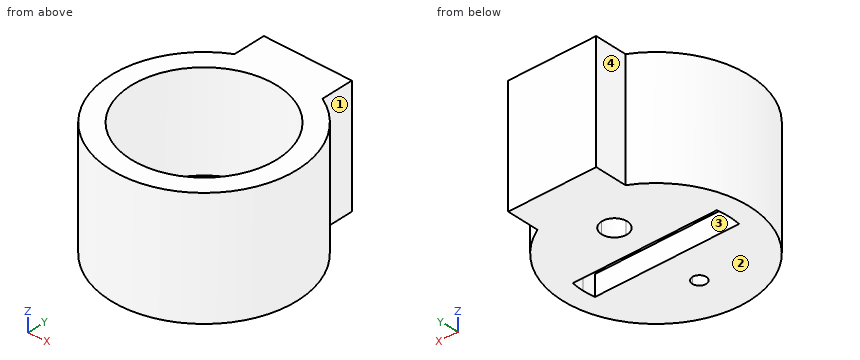
from build123d import *

# Parameters (mm, degrees)
F0_W     = 330
F0_H     = 300
F1_DEPTH = 110
F2_R     = 68.5
F3_DEPTH = 90.8
F5_DEPTH = 19.201
F2_W     = 330
F2_H     = 300
F2_R_2   = 87.5
F6_DEPTH = 110.001
F8_DEPTH = 110


with BuildPart() as f1:
    # F0 (on Top) → F1 (new body)
    with BuildSketch(Plane.XY):
        Rectangle(F0_W, F0_H)
    extrude(amount=-F1_DEPTH)

    # F2 (on Top) → F3 (cut)
    with BuildSketch(Plane.XY):
        Circle(F2_R)
    extrude(amount=-F3_DEPTH, mode=Mode.SUBTRACT)

    # F4 (on face) → F5 (cut, through all)
    with BuildSketch(Plane.XY.offset(-90.8)):
        with BuildLine():
            Line((0, -11.5), (0, 0))
            Line((0, 0), (0, 11.5))
            Line((0, 11.5), (-67.5277720645, 11.5))
            ThreePointArc((-67.5277720645, 11.5), (-68.5, 0), (-67.5277720645, -11.5))
            Line((-67.5277720645, -11.5), (0, -11.5))
        make_face()
        with BuildLine():
            Line((0, 11.5), (0, 0))
            Line((0, 0), (0, -11.5))
            Line((0, -11.5), (67.5277720645, -11.5))
            ThreePointArc((67.5277720645, -11.5), (68.2565102625, -5.7705118308), (68.5, 0))
            ThreePointArc((68.5, 0), (68.2565102625, 5.7705118308), (67.5277720645, 11.5))
            Line((67.5277720645, 11.5), (0, 11.5))
        make_face()
        with BuildLine():
            ThreePointArc((12, 43), (-8.4852813742, 51.4852813742), (0, 31))
            ThreePointArc((0, 31), (8.4852813742, 34.5147186258), (12, 43))
        make_face()
        with BuildLine():
            ThreePointArc((6.5, -45), (4.5961940777, -40.4038059223), (0, -38.5))
            ThreePointArc((0, -38.5), (-4.5961940777, -49.5961940777), (6.5, -45))
        make_face()
    extrude(amount=-F5_DEPTH, mode=Mode.SUBTRACT)

    # F2 (on Top) → F6 (cut, through all)
    with BuildSketch(Plane.XY):
        Rectangle(F2_W, F2_H)
        Circle(F2_R_2, mode=Mode.SUBTRACT)
    extrude(amount=-F6_DEPTH, mode=Mode.SUBTRACT)

    # F7 (on face) → F8 (join)
    with BuildSketch(Plane(origin=(0, 0, -110), x_dir=(1, 0, 0), z_dir=(0, 0, -1))):
        with BuildLine():
            ThreePointArc((41.25, -77.1666216703), (0, -87.5), (-41.25, -77.1666216703))
            Line((-41.25, -77.1666216703), (-41.25, -107.5))
            Line((-41.25, -107.5), (41.25, -107.5))
            Line((41.25, -107.5), (41.25, -77.1666216703))
        make_face()
    extrude(amount=-F8_DEPTH)


solid = f1.part
Design review of the part built by this model. Coordinates are the model's own, in mm. Face numbers are marked on the shaded views. Round coordinates to 2 decimals unless told otherwise and drop trailing zeros. Write each loop counter-clockwise with the first axis right and the second up, starting at its lowest first coordinate (ties: lowest second). Pieces come first, ordered by that corner, then holes. Notation, with made-up numbers: (9.25, -29) - (20.25, -29) arc R20 ccw to (20.25, -5) - close; hole circle Ø2 at (1.5, 57.25). An arc over 180 degrees is marked (long way). Use a Markdown table: item, result. Add a question column.
1. We need section C-C (z = -7.5). State the section outline as (x, y) points.
2. We need section D-D (y = -56). State the section outline as (x, z) points.
3. We need section B-B (y = -7). State the section outline as (x, z) points.
4. Wall thickness on probe 1 along Y at (x, z) = (0, -105.5); probe 2 along Y at (x, z) = (0, -36); probe 3 along Z at (x, y) = (37.5, -28.5): over which ranges is each line inside the solid? List them lowest first.
5. Clearance check with flat-ended pins moving along their axes: pin 1 (21 mm diameter, centred on x = 31, z = -101.5, fed in from -Y); pin 2 (5 mm diameter, centred on x = -31.5, z = -33, fed in from -Y); pin 3 (10 mm diameter, centred on x = 58, z = -33, fed in from +Y); pin 4 (10.5 mm diameter, centred on x = 0, y = -45, fed in from -Z). State where each tip first meets the part, or that it passes through.
6. Mouldability with a two-part tool opening along X and no side actions: class the marked faces 1, 2, 3 and 4 as +X half, -X half, draft (parallel to the pull), parting line (faces both ways), or undercut.
7. We need section A-A (z = -98). State the section outline as (x, y) points.
Output:
| question | item | result |
|---|---|---|
| 1 | outline | (-41.25, 77.17) arc R87.5 ccw (long way) to (41.25, 77.17) - (41.25, 107.5) - (-41.25, 107.5) - close; hole circle Ø137 at (0, 0) |
| 2 | outline | (-67.23, -110) - (67.23, -110) - (67.23, 0) - (39.45, 0) - (39.45, -90.8) - (-39.45, -90.8) - (-39.45, 0) - (-67.23, 0) - close |
| 3 | outline | (-87.22, -110) - (-68.14, -110) - (-68.14, 0) - (-87.22, 0) - close; (68.14, -110) - (87.22, -110) - (87.22, 0) - (68.14, 0) - close |
| 4 | probe 1 | y = -87.5 to -51.5, -38.5 to -11.5, 11.5 to 31, 55 to 107.5 |
| 4 | probe 2 | y = -87.5 to -68.5, 68.5 to 107.5 |
| 4 | probe 3 | z = -110 to -90.8 |
| 5 | pin 1 | stops at y = -85.06 |
| 5 | pin 2 | stops at y = -82.55 |
| 5 | pin 3 | stops at y = 69.62 |
| 5 | pin 4 | passes through |
| 6 | face 1 | +X half |
| 6 | face 2 | draft |
| 6 | face 3 | undercut |
| 6 | face 4 | -X half |
| 7 | outline | (-41.25, 77.17) arc R87.5 ccw (long way) to (41.25, 77.17) - (41.25, 107.5) - (-41.25, 107.5) - close; hole (-67.53, -11.5) - (67.53, -11.5) arc R68.5 ccw to (67.53, 11.5) - (-67.53, 11.5) arc R68.5 ccw to start; hole circle Ø24 at (0, 43); hole circle Ø13 at (0, -45) |
